Autodesk Inventor part; units mm, degrees
ref_plane "YZ Plane" through (0, 0, 0) normal (1, 0, 0) x (0, 1, 0)
ref_plane "XZ Plane" through (0, 0, 0) normal (0, 1, 0) x (-1, 0, 0)
ref_plane "XY Plane" through (0, 0, 0) normal (0, 0, 1) x (1, 0, 0)
sketch "スケッチ1" plane through (0, 0, 0) normal (0, 0, 1) x (1, 0, 0)
  line L0 (0, 0) -> (-20.5, 0)
  line L1 (-20.5, 0) -> (-20.5, -17)
  line L2 (-20.5, -17) -> (0, -17)
  line L3 (0, -17) -> (0, 0)
  dimension "d0" = 20.5
  dimension "d1" = 17
extrude "押し出し1" add sketch "スケッチ1" along normal blind 4
sketch "スケッチ2" plane through (0, 0, 4) normal (0, 0, 1) x (1, 0, 0)
  circle A0 centre (-5.5, -2.5) radius 0.8
  circle A1 centre (-5.5, -14.5) radius 0.8
  point P0 (0, 0)
  dimension "d4" = 1.6
  dimension "d5" = 1.6
extrude "押し出し2" cut sketch "スケッチ2" against normal blind 4
sketch "スケッチ3" plane through (0, 0, 4) normal (0, 0, 1) x (1, 0, 0)
  line L0 (0, -17) -> (0, 0)
  line L1 (0, -8.5) -> (0, -11.6)
  line L2 (0, -11.6) -> (-18.5, -11.6)
  line L3 (-20.5, 0) -> (-20.5, -17)
  line L4 (-18.5, -11.6) -> (-18.5, -5.4)
  line L5 (-18.5, -5.4) -> (0, -5.4)
  line L6 (0, -5.4) -> (0, -8.5)
  point P0 (0, -5.4)
  dimension "d8" = 3.1
  dimension "d9" = 18.5
  dimension "d10" = 6.2
extrude "押し出し3" cut sketch "スケッチ3" against normal blind 0.7
sketch "スケッチ4" plane through (0, 0, 3.3) normal (0, 0, 1) x (1, 0, 0)
  circle A0 centre (-13.25, -8.5) radius 1.2
  circle A1 centre (-10.846154, -8.5) radius 1.203846
  line L0 (-10.75, -9.7) -> (-13.25, -9.7)
  line L1 (-10.75, -7.3) -> (-13.25, -7.3)
  line L2 (-18.5, -11.6) -> (-18.5, -5.4)
  point P0 (0, 0)
  dimension "d13" = 2.4
  dimension "d16" = 5.25
  dimension "d17" = 2.5
sketch "スケッチ4 outline for 押し出し4" plane through (0, 0, 3.3) normal (0, 0, 1) x (1, 0, 0)
  line L0 (-13.25, -9.7) -> (-10.75, -9.7)
  arc A0 (-13.25, -7.3) -> (-13.25, -9.7) centre (-13.25, -8.5) ccw
  line L1 (-10.75, -7.3) -> (-13.25, -7.3)
  arc A1 (-10.75, -9.7) -> (-10.75, -7.3) centre (-10.846154, -8.5) ccw
extrude "押し出し4" add sketch "スケッチ4 outline for 押し出し4" along normal blind 0.7
sketch "スケッチ5" plane through (0, 0, 4) normal (0, 0, 1) x (1, 0, 0)
  line L0 (-20.5, -17) -> (-20.5, -12)
  line L1 (-20.5, -17) -> (-16.5, -17)
  line L2 (-20.5, 0) -> (-20.5, -5)
  line L3 (-20.5, 0) -> (-16.5, 0)
  line L4 (0, 0) -> (-20.5, 0)
  line L5 (-16.5, 0) -> (-20.5, -5)
  dimension "d18" = 5
  dimension "d19" = 4
  dimension "d20" = 5
  dimension "d21" = 4
extrude "押し出し5" cut sketch "スケッチ5" against normal blind 10
fillet "フィレット1" radius 2 5 edges at (-16.5, 0, 2) (-20.5, -5, 2) (-20.5, -17, 2) (0, -17, 2) (0, 0, 2)
fillet_without_effect "フィレット2"
sketch "スケッチ6" plane through (0, 0, 3.3) normal (0, 0, 1) x (1, 0, 0)
  line L0 (-18.5, -5.4) -> (0, -5.4)
  circle A0 centre (-18, -5.9) radius 0.707107
  line L1 (0, -11.6) -> (-18.5, -11.6)
  circle A1 centre (-18, -11.1) radius 0.707107
  line L2 (-18.5, -11.6) -> (-18.5, -5.4)
  point P0 (0, 0)
  dimension "d28" = 0.5
  dimension "d29" = 0.5
  dimension "d30" = 0.5
  dimension "d31" = 0.5
extrude "押し出し6" cut sketch "スケッチ6" along normal blind 0.7
properties part number "cutter_holder-2" material "ABS プラスチック"
Read the model definition and answer for the solid it produces. Units are mm, in the model's axes. A direction names the side the tool comes from. Give positions to 0.01 mm unless a question says otherwise; leave off trailing zeros. Loops run counter-clockwise (first coordinate to the right, second up) from the corner with the lowest first, then second, coordinate; pieces in that order, holes last. Notation, with made-up numbers: (24, -31) -> (43, -31) arc R27 ccw to (43, -10) -> close; hole circle Ø7 at (-7.5, 49). An arc over 180 degrees is marked (long way). Use a Markdown table: item, result.
Q1. Section C-C, the plane z = 1.65 is taken. Determine the outline of the cut face in (x, y).
Solved:
| item | result |
|---|---|
| outline | (-20.5, -15) arc R2 ccw to (-18.5, -17) -> (-2, -17) arc R2 ccw to (0, -15) -> (0, -2) arc R2 ccw to (-2, 0) -> (-15.54, 0) arc R2 ccw to (-17.1, -0.75) -> (-20.06, -4.45) arc R2 ccw to (-20.5, -5.7) -> close; hole circle Ø1.6 at (-5.5, -14.5); hole circle Ø1.6 at (-5.5, -2.5) |
Q2. Section D-D, the plane x = -8.5 is taken. Determine the outline of the cut face in (y, z), then the cut area to 3 significant figures.
Solved:
| item | result |
|---|---|
| outline | (-17, 0) -> (0, 0) -> (0, 4) -> (-5.4, 4) -> (-5.4, 3.3) -> (-11.6, 3.3) -> (-11.6, 4) -> (-17, 4) -> close |
| area | 63.7 mm^2 |
Q3. Find the intervals of material crossed by line 1 along Y through (x, z) = (-5.5, 3.2); line 2 along X through (y, z) = (-2.25, 2.9); line 3 along Z through (x, y) = (-10.25, -6.5), in increasing order.
Solved:
| item | result |
|---|---|
| line 1 | y = -17 to -15.3, -13.7 to -3.3, -1.7 to 0 |
| line 2 | x = -18.3 to -6.26, -4.74 to 0 |
| line 3 | z = 0 to 3.3 |
Q4. This flat-tipped pin is pushed along its axis until it touches: pin 1 (1 mm diameter, centred on y = -6.5, z = 0.5, fed in from +X). Where does it stop, or does it pass through?
Solved:
| item | result |
|---|---|
| pin 1 | stops at x = 0 |
Q5. Section B-B, the plane x = -5.5 is taken. Determine the outline of the cut face in (y, z), then the cut area to 3 significant figures.
Solved:
| item | result |
|---|---|
| outline | (-17, 0) -> (-15.3, 0) -> (-15.3, 4) -> (-17, 4) -> close; (-13.7, 0) -> (-3.3, 0) -> (-3.3, 4) -> (-5.4, 4) -> (-5.4, 3.3) -> (-11.6, 3.3) -> (-11.6, 4) -> (-13.7, 4) -> close; (-1.7, 0) -> (0, 0) -> (0, 4) -> (-1.7, 4) -> close |
| area | 50.9 mm^2 |
Q6. Section A-A, the plane y = -2.5 is taken. Determine the outline of the cut face in (x, z), then the cut area to 3 significant figures.
Solved:
| item | result |
|---|---|
| outline | (-18.5, 0) -> (-6.3, 0) -> (-6.3, 4) -> (-18.5, 4) -> close; (-4.7, 0) -> (0, 0) -> (0, 4) -> (-4.7, 4) -> close |
| area | 67.6 mm^2 |
Q7. Determine the mould class of faces 4 (the face through (-18.56, -2.575, 2.028)), 5 (the face through (-20.5, -10, 2)), 6 (the face through (-18.5, -11.6, 3.6)), 7 (the face through (-10, -17, 2)) for opening direction Y: pulls with the +Y half, pulls with the -Y half, needs draft (parallel to the pull), parting line crosses it, or undercut.
Solved:
| item | result |
|---|---|
| face 4 | pulls with the +Y half |
| face 5 | needs draft |
| face 6 | undercut |
| face 7 | pulls with the -Y half |
Q8. A tool of negligible diameter and unlimited length cuts with its end or side. For faces 1 (the face through (-18.5, -5.4, 3.6)), 2 (the face through (-10, -12, 4)), 3 (the face through (-9.643, -8.475, 3.645)), from which of +Z, -Z, +X, -X, +Y, -Y can it reach the whole face along a straight path? Write none if from no direction.
Solved:
| item | result |
|---|---|
| face 1 | +Z |
| face 2 | +Z, +X, -X, +Y, -Y |
| face 3 | +Z, +X |
